```python
from build123d import *

# Parameters (mm, degrees)
BOSS_EXTRUDE2_DEPTH = 135
SKETCH2_R           = 20
SKETCH2_W           = 100
SKETCH2_H           = 20
BOSS_EXTRUDE3_DEPTH = 30
SKETCH3_W           = 84.902161113
SKETCH3_H           = 18.014954353
CUT_EXTRUDE1_DEPTH  = 30
FILLET1_R           = 10
FILLET2_R           = 10


with BuildPart() as part:
    # Sketch1 → Boss-Extrude2 (new body)
    with BuildSketch(Plane.XY):
        with BuildLine():
            Line((-21.469266172, 234.360279406), (153.530733828, 234.360279406))
            Line((153.530733828, 234.360279406), (158.530733828, 194.360279406))
            Line((158.530733828, 194.360279406), (158.530733828, 14.360279406))
            ThreePointArc((158.530733828, 14.360279406), (143.886072887, -20.995059653), (108.530733828, -35.639720594))
            Line((108.530733828, -35.639720594), (23.530733828, -35.639720594))
            ThreePointArc((23.530733828, -35.639720594), (-11.824605232, -20.995059653), (-26.469266172, 14.360279406))
            Line((-26.469266172, 14.360279406), (-26.469266172, 194.360279406))
            Line((-26.469266172, 194.360279406), (-21.469266172, 234.360279406))
        make_face()
    extrude(amount=BOSS_EXTRUDE2_DEPTH)

    # Sketch2 → Boss-Extrude3 (add)
    with BuildSketch(Plane(origin=(0, 234.360279406, 0), x_dir=(1, 0, 0), z_dir=(0, 1, 0))):
        with Locations(Location((-1.469266172, -67.5, 0), (0, 0, 180))):
            Circle(SKETCH2_R)
        with Locations((86.735726722, -67.5)):
            Rectangle(SKETCH2_W, SKETCH2_H)
    extrude(amount=BOSS_EXTRUDE3_DEPTH)

    # Sketch3 → Cut-Extrude1 (cut)
    with BuildSketch(Plane.XY.offset(77.5)):
        with Locations((86.110215993, 249.037763676)):
            Rectangle(SKETCH3_W, SKETCH3_H)
    extrude(amount=-CUT_EXTRUDE1_DEPTH, mode=Mode.SUBTRACT)

    # Fillet1
    fillet1_edges = [part.edges().sort_by_distance(p)[0] for p in [
        (158.530733828, 104.360279406, 135),
        (143.886072887, -20.995059653, 135),
        (66.030733828, -35.639720594, 135),
        (-11.824605232, -20.995059653, 135),
        (-26.469266172, 104.360279406, 135),
    ]]
    fillet(fillet1_edges, radius=FILLET1_R)

    # Fillet2
    # the kernel refuses this fillet: 10 mm, written as the material it takes off along each edge
    with BuildSketch(Plane(origin=(-26.469266172, 14.360279406, 0), x_dir=(0, 0, 1), z_dir=(0, 1, 0))) as fillet2_piece_1:
        with BuildLine():
            CenterArc((FILLET2_R, FILLET2_R), FILLET2_R, 180, 90)
            Line((0, FILLET2_R), (-FILLET2_R * 0.02, FILLET2_R))
            Line((-FILLET2_R * 0.02, FILLET2_R), (-FILLET2_R * 0.02, -FILLET2_R * 0.02))
            Line((-FILLET2_R * 0.02, -FILLET2_R * 0.02), (FILLET2_R, -FILLET2_R * 0.02))
            Line((FILLET2_R, -FILLET2_R * 0.02), (FILLET2_R, 0))
        make_face()
    extrude(amount=240, mode=Mode.SUBTRACT)
    with BuildSketch(Plane(origin=(23.530733828, 14.360279406, 0), x_dir=(0, -1, 0), z_dir=(1, 0, 0))) as fillet2_piece_2:
        with BuildLine():
            CenterArc((50 - FILLET2_R, -FILLET2_R), FILLET2_R, 0, 90)
            Line((50 - FILLET2_R, 0), (50 - FILLET2_R, FILLET2_R * 0.02))
            Line((50 - FILLET2_R, FILLET2_R * 0.02), (50 + FILLET2_R * 0.02, FILLET2_R * 0.02))
            Line((50 + FILLET2_R * 0.02, FILLET2_R * 0.02), (50 + FILLET2_R * 0.02, -FILLET2_R))
            Line((50 + FILLET2_R * 0.02, -FILLET2_R), (50, -FILLET2_R))
        make_face()
    revolve(axis=Axis((23.530733828, 14.360279406, 0), (0, 0, -1)), revolution_arc=90, mode=Mode.SUBTRACT)
    with BuildSketch(Plane(origin=(108.530733828, -35.639720594, 0), x_dir=(0, 1, 0), z_dir=(-1, 0, 0))) as fillet2_piece_3:
        with BuildLine():
            CenterArc((FILLET2_R, -FILLET2_R), FILLET2_R, 90, 90)
            Line((0, -FILLET2_R), (-FILLET2_R * 0.02, -FILLET2_R))
            Line((-FILLET2_R * 0.02, -FILLET2_R), (-FILLET2_R * 0.02, FILLET2_R * 0.02))
            Line((-FILLET2_R * 0.02, FILLET2_R * 0.02), (FILLET2_R, FILLET2_R * 0.02))
            Line((FILLET2_R, FILLET2_R * 0.02), (FILLET2_R, 0))
        make_face()
    extrude(amount=85, mode=Mode.SUBTRACT)
    with BuildSketch(Plane(origin=(108.530733828, 14.360279406, 0), x_dir=(1, 0, 0), z_dir=(0, 1, 0))) as fillet2_piece_4:
        with BuildLine():
            CenterArc((50 - FILLET2_R, -FILLET2_R), FILLET2_R, 0, 90)
            Line((50, -FILLET2_R), (50 + FILLET2_R * 0.02, -FILLET2_R))
            Line((50 + FILLET2_R * 0.02, -FILLET2_R), (50 + FILLET2_R * 0.02, FILLET2_R * 0.02))
            Line((50 + FILLET2_R * 0.02, FILLET2_R * 0.02), (50 - FILLET2_R, FILLET2_R * 0.02))
            Line((50 - FILLET2_R, FILLET2_R * 0.02), (50 - FILLET2_R, 0))
        make_face()
    revolve(axis=Axis((108.530733828, 14.360279406, 0), (0, 0, -1)), revolution_arc=90, mode=Mode.SUBTRACT)
    with BuildSketch(Plane(origin=(158.530733828, 254.360279406, 0), x_dir=(-1, 0, 0), z_dir=(0, -1, 0))) as fillet2_piece_5:
        with BuildLine():
            CenterArc((FILLET2_R, -FILLET2_R), FILLET2_R, 90, 90)
            Line((0, -FILLET2_R), (-FILLET2_R * 0.02, -FILLET2_R))
            Line((-FILLET2_R * 0.02, -FILLET2_R), (-FILLET2_R * 0.02, FILLET2_R * 0.02))
            Line((-FILLET2_R * 0.02, FILLET2_R * 0.02), (FILLET2_R, FILLET2_R * 0.02))
            Line((FILLET2_R, FILLET2_R * 0.02), (FILLET2_R, 0))
        make_face()
    extrude(amount=240, mode=Mode.SUBTRACT)


solid = part.part
```
Input: part model. Units: mm. Frame: model coordinates. A direction names the side the tool comes from. Coordinates: 2 decimals unless noted, no trailing zeros. Loops run counter-clockwise (first coordinate to the right, second up) from the corner with the lowest first, then second, coordinate; pieces in that order, holes last. Notation, with made-up numbers: M -22,5 L -15,5 A33 ccw -15,40 Z; hole C 76,10 d3. An arc over 180 degrees is marked long. One line per item, written item: value.
(1) Section D-D (y = 228). Output: boundary loops of the cut face in (x, z), and give its area (3 significant figures).
Filled in:
outline: M -22.26,1.85 A10 ccw -16.47,0 L 148.53,0 A10 ccw 154.33,1.85 L 154.33,133.15 A10 ccw 148.53,135 L -16.47,135 A10 ccw -22.26,133.15 Z
area: 23,800 mm^2
(2) Pull-direction query (X, two-part tool) for faces 4 (the flat face through (67, 106, 0)), 5 (the flat face through (86, 258.045, 68)), 6 (the cylindrical face through (-23.46, 125.9, 132.15)), 7 (the flat face through (136.736, 249, 68)); classes: +X half, -X half, draft (parallel to the pull), parting line (faces both ways), or undercut.
Filled in:
face 4: draft
face 5: undercut
face 6: -X half
face 7: +X half
(3) Line query: line 1 along Y through (x, z) = (51, 69); line 2 along Y through (x, z) = (48.5, 115); line 3 along Y through (x, z) = (-1.5, 70). Output: solid intervals per line, ascending. Write a range as from..to.
Filled in:
line 1: -35.64..240.03, 258.05..264.36
line 2: -35.64..234.36
line 3: -28.92..264.36
(4) Pin query (flat end, axial travel): pin 1 (10 mm diameter, centred on y = 255.5, z = 67, fed in from +X); pin 2 (24 mm diameter, centred on x = 93, y = 248, fed in from -Z); pin 3 (3 mm diameter, centred on y = -1.5, z = 102, fed in from -X); pin 4 (15 mm diameter, centred on x = 70.5, y = 249.5, fed in from +Z). Return the tip coordinate at first contact, or that it passes through.
Filled in:
pin 1: x = 136.74
pin 2: z = 57.5
pin 3: x = -24.36
pin 4: through
(5) Reachability of faces 1 (the flat face through (86, 239, 77.5)), 2 (the cylindrical face through (2.866, 249.15, 47.976)), 3 (the flat face through (43.659, 249, 68)) from +Z, -Z, +X, -X, +Y, -Y: full face, straight path, thin tool, end or side. Return the list, or none.
Filled in:
face 1: +Z, +X, +Y
face 2: +Y
face 3: +Z, -Z
(6) Section C-C (x = 33.5). Output: boundary loops of the cut face in (y, z).
Filled in:
outline: M -35.64,10 A10 ccw -25.64,0 L 234.36,0 L 234.36,135 L -25.64,135 A10 ccw -35.64,125 Z
(7) Section B-B (z = 97.5). Output: boundary loops of the cut face in (x, y), and give its area (3 significant figures).
Filled in:
outline: M -26.47,14.36 A50 ccw 23.53,-35.64 L 108.53,-35.64 A50 ccw 158.53,14.36 L 158.53,194.36 L 153.53,234.36 L -21.47,234.36 L -26.47,194.36 Z
area: 48,700 mm^2
(8) Section A-A (x = 101). Output: boundary loops of the cut face in (y, z), and give its area (3 significant figures).
Filled in:
outline: M -35.64,10 A10 ccw -25.64,0 L 234.36,0 L 234.36,57.5 L 240.03,57.5 L 240.03,77.5 L 234.36,77.5 L 234.36,135 L -25.64,135 A10 ccw -35.64,125 Z; M 258.05,57.5 L 264.36,57.5 L 264.36,77.5 L 258.05,77.5 Z
area: 36,600 mm^2
